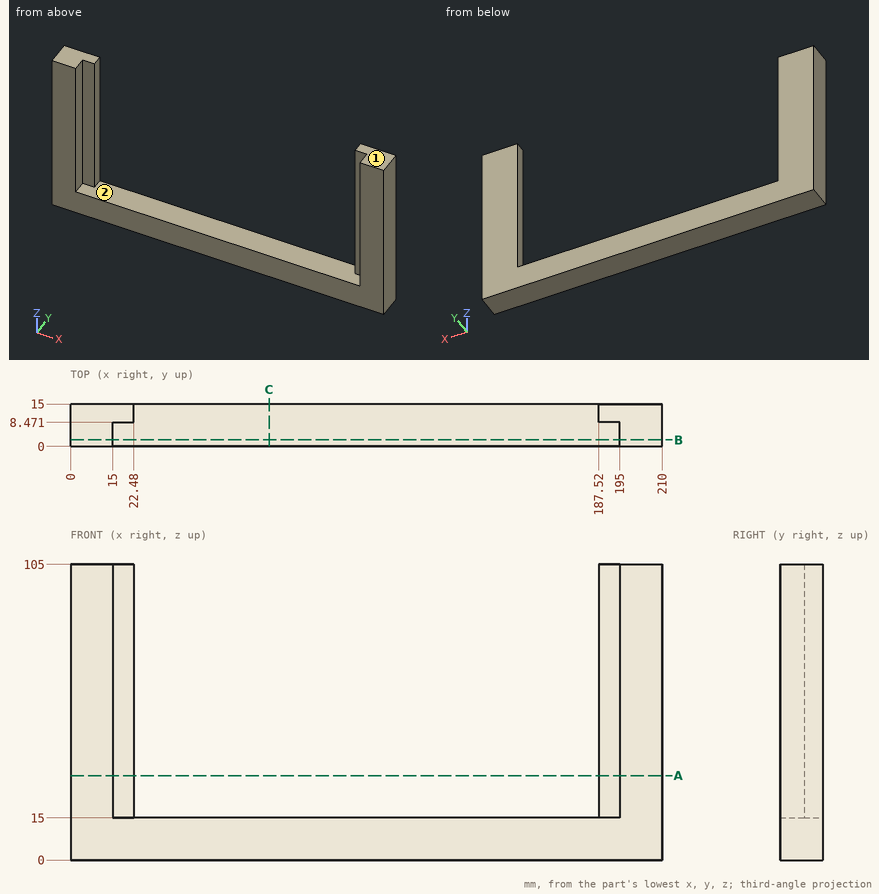
The drawing under review shows one solid part. Ordinate dimensions are in mm from its lowest x, y, z. Coordinates: 2 decimals unless noted, no trailing zeros. Write each loop counter-clockwise with the first axis right and the second up, starting at its lowest first coordinate (ties: lowest second). Pieces come first, ordered by that corner, then holes. Notation, with made-up numbers: M -14.5,-33.5 L 24.5,-33.5 A18 ccw 24.5,-13.5 Z; hole C 78,77.25 d5. An arc over 180 degrees is marked long. Put each result on its own line as item: value.
1) Clearance check with flat-ended pins moving along their axes: pin 1 Ø7.5 at (x, y) = (142, 9.5) entering from +Z; pin 2 Ø2 at (x, z) = (192.5, 40.5) entering from -Y. State where each tip first meets the part, or that it passes through.
Computed:
pin 1: stops at z = 15
pin 2: stops at y = 8.47
2) Add section A-A on z = 30. Give the boundary of the cut face in (x, y), then the cut area to 3 significant figures.
Computed:
outline: M 0,0 L 15,0 L 15,8.47 L 22.48,8.47 L 22.48,15 L 0,15 Z; M 187.52,8.47 L 195,8.47 L 195,0 L 210,0 L 210,15 L 187.52,15 Z
area: 548 mm2
3) Wall thickness on probe 1 along X at (y, z) = (1.25, 50); probe 2 along X at (y, z) = (11.5, 73); probe 3 along Z at (x, y) = (101, 10): over which ranges is each line inside the solid? List them lowest first. Write a range as [from, to].
Computed:
probe 1: x = [0, 15], [195, 210]
probe 2: x = [0, 22.48], [187.52, 210]
probe 3: z = [0, 15]
4) Draft analysis for pull direction X (two halves, no side actions). For the marked faces 1 and 2, state which applies: released by +X, released by -X, zero draft, split by the parting line, or undercut.
Computed:
face 1: zero draft
face 2: undercut
5) Add section B-B on y = 2.25. Give the boundary of the cut face in (x, z).
Computed:
outline: M 0,0 L 210,0 L 210,105 L 195,105 L 195,15 L 15,15 L 15,105 L 0,105 Z
6) Add section C-C on x = 70.5. Give the boundary of the cut face in (y, z).
Computed:
outline: M 0,0 L 15,0 L 15,15 L 0,15 Z
